Can you work these out from the model? Positions are in its coordinate system, mm. Give positions to 0.01 mm unless a question says otherwise; leave off trailing zeros. Order: outer loops, then holes, each group sorted by start corner. A loop starts at its lowest first (then second) coordinate and runs counter-clockwise, first axis right, second up.
Item 1: I'm going to push a flat-ended pin straight in: pin 1 Ø6 at (x, y) = (3.5, 12.5) entering from -Z. Where does the tip first touch, or does it pass through?
Item 2: I want a section at B-B, the plane x = 2.75. Count the separate pieces of the cut face and the enclosed holes in it, then the cut area to 3 significant figures.
Item 3: I want a section at A-A, the plane y = 13.5. Write out the boundary of the cut face in (x, z).
Item 4: If I drill on line 1 along X through (y, z) = (16, 0.05); line 2 along X through (y, z) = (4, 0.25), over which ranges is the centre line in solid material (lowest first)?
Item 5: I want a section at C-C, the plane y = 16.5. Write out the boundary of the cut face in (x, z).
```python
from build123d import *

# Parameters (mm, degrees)
SKETCH_1_W             = 12.5
SKETCH_1_H             = 0.5
EXTRUDE_1_DEPTH        = 0.4
PATTERN_LINEAR_1_COUNT = 7
PATTERN_LINEAR_1_PITCH = 2.5
EXTRUDE_3_DEPTH        = 0.4
PATTERN_LINEAR_2_COUNT = 7
PATTERN_LINEAR_2_PITCH = 2.5
SKETCH_4_W             = 0.5
SKETCH_4_H             = 2.5
EXTRUDE_4_DEPTH        = 0.4
SKETCH_6_W             = 0.5
SKETCH_6_H             = 2.5
EXTRUDE_6_DEPTH        = 0.4
SKETCH_7_W             = 10.5
SKETCH_7_H             = 0.5
SKETCH_7_W_2           = 5.5
EXTRUDE_7_DEPTH        = 0.4
CUT_EXTRUDE_2_DEPTH    = 10


with BuildPart() as part:
    # Sketch 1 → Extrude 1 (new body)
    with BuildSketch(Plane.XY):
        with Locations((6.25, 0.25)):
            Rectangle(SKETCH_1_W, SKETCH_1_H)
    extrude(amount=EXTRUDE_1_DEPTH)


with BuildPart() as pattern_linear_1_1:
    # Pattern Linear 1: pattern copy
    add(part.part.moved(Location(Vector(0, 1, 0) * (1 * PATTERN_LINEAR_1_PITCH))))


with BuildPart() as pattern_linear_1_2:
    # Pattern Linear 1: pattern copy
    add(part.part.moved(Location(Vector(0, 1, 0) * (2 * PATTERN_LINEAR_1_PITCH))))


with BuildPart() as pattern_linear_1_3:
    # Pattern Linear 1: pattern copy
    add(part.part.moved(Location(Vector(0, 1, 0) * (3 * PATTERN_LINEAR_1_PITCH))))


with BuildPart() as pattern_linear_1_4:
    # Pattern Linear 1: pattern copy
    add(part.part.moved(Location(Vector(0, 1, 0) * (4 * PATTERN_LINEAR_1_PITCH))))


with BuildPart() as pattern_linear_1_5:
    # Pattern Linear 1: pattern copy
    add(part.part.moved(Location(Vector(0, 1, 0) * (5 * PATTERN_LINEAR_1_PITCH))))


with BuildPart() as pattern_linear_1_6:
    # Pattern Linear 1: pattern copy
    add(part.part.moved(Location(Vector(0, 1, 0) * (6 * PATTERN_LINEAR_1_PITCH))))

    # Sketch 4 → Extrude 4 (add)
    with BuildSketch(Plane.XY.offset(0.4)):
        with Locations((4.75, 16.75)):
            Rectangle(SKETCH_4_W, SKETCH_4_H)
        with Locations((2.25, 16.75)):
            Rectangle(SKETCH_4_W, SKETCH_4_H)
        with Locations((7.25, 16.75)):
            Rectangle(SKETCH_4_W, SKETCH_4_H)
        with Locations((9.75, 16.75)):
            Rectangle(SKETCH_4_W, SKETCH_4_H)
    extrude(amount=-EXTRUDE_4_DEPTH)

    # Sketch 6 → Extrude 6 (add)
    with BuildSketch(Plane.XY.offset(0.4)):
        with Locations((4.75, 19.25)):
            Rectangle(SKETCH_6_W, SKETCH_6_H)
        with Locations((9.75, 19.25)):
            Rectangle(SKETCH_6_W, SKETCH_6_H)
        with Locations((7.25, 19.25)):
            Rectangle(SKETCH_6_W, SKETCH_6_H)
    extrude(amount=-EXTRUDE_6_DEPTH)

    # Sketch 7 → Extrude 7 (add)
    with BuildSketch(Plane.XY.offset(0.4)):
        with Locations((7.25, 17.75)):
            Rectangle(SKETCH_7_W, SKETCH_7_H)
        with Locations((7.25, 20.25)):
            Rectangle(SKETCH_7_W_2, SKETCH_7_H)
    extrude(amount=-EXTRUDE_7_DEPTH)

    # Sketch 9 → Cut-Extrude 2 (cut)
    with BuildSketch(Plane.XY.offset(0.4)):
        Polygon((9.5, 18), (10, 18), (10, 15.5), (12.5, 15.5), (12.5, 20), (10, 20), (10, 20.5), (7.5, 20.5), (7.5, 20), (9.5, 20), align=None)
    extrude(amount=-CUT_EXTRUDE_2_DEPTH, mode=Mode.SUBTRACT)


with BuildPart() as part_1:
    add(part.part)

    add(pattern_linear_1_1.part)  # Extrude 3 merges Pattern Linear 1_1

    add(pattern_linear_1_2.part)  # Extrude 3 merges Pattern Linear 1_2

    add(pattern_linear_1_3.part)  # Extrude 3 merges Pattern Linear 1_3
    # Sketch 3 → Extrude 3 (add)
    with BuildSketch(Plane.XY.offset(0.4)):
        Polygon((0, 15.5), (0, 8), (0, 0), (-0.5, 0), (-0.5, 10.98507125), (-0.5, 15.5), align=None)
    extrude_3 = extrude(amount=-EXTRUDE_3_DEPTH)

    # Pattern Linear 2: Extrude 3 ×7, 1 skipped
    with Locations(*[(i * PATTERN_LINEAR_2_PITCH, 0, 0) for i in range(1, PATTERN_LINEAR_2_COUNT) if i not in (6,)]):
        add(extrude_3)

    # Combine 1: union Pattern Linear 1_5, Pattern Linear 1_4
    add(pattern_linear_1_5.part)
    add(pattern_linear_1_4.part)

    # Combine 2: union Pattern Linear 1_6
    add(pattern_linear_1_6.part)


solid = part_1.part
```
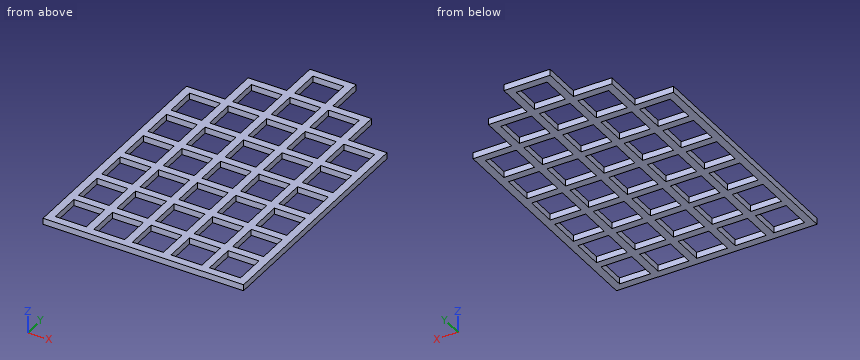
Results list:
1. pin 1: stops at z = 0
2. separate pieces: 8
2. enclosed holes: 0
2. area: 1.60 mm2
3. outline: (-0.5, 0) - (0, 0) - (0, 0.4) - (-0.5, 0.4) - close; (2, 0) - (2.5, 0) - (2.5, 0.4) - (2, 0.4) - close; (4.5, 0) - (5, 0) - (5, 0.4) - (4.5, 0.4) - close; (7, 0) - (7.5, 0) - (7.5, 0.4) - (7, 0.4) - close; (9.5, 0) - (10, 0) - (10, 0.4) - (9.5, 0.4) - close; (12, 0) - (12.5, 0) - (12.5, 0.4) - (12, 0.4) - close
4. line 1: x = 2 to 2.5, 4.5 to 5, 7 to 7.5, 9.5 to 10
4. line 2: x = -0.5 to 0, 2 to 2.5, 4.5 to 5, 7 to 7.5, 9.5 to 10, 12 to 12.5
5. outline: (2, 0) - (2.5, 0) - (2.5, 0.4) - (2, 0.4) - close; (4.5, 0) - (5, 0) - (5, 0.4) - (4.5, 0.4) - close; (7, 0) - (7.5, 0) - (7.5, 0.4) - (7, 0.4) - close; (9.5, 0) - (10, 0) - (10, 0.4) - (9.5, 0.4) - close
